The model under review builds one solid part; all positions refer to its coordinate system, in mm. A direction names the side the tool comes from. Give positions to 0.01 mm unless a question says otherwise; leave off trailing zeros. Write each loop counter-clockwise with the first axis right and the second up, starting at its lowest first coordinate (ties: lowest second). Pieces come first, ordered by that corner, then holes. Notation, with made-up numbers: M -37.75,-9 L -14.75,-9 A21 cw -14.75,30 Z; hole C -28,22.5 d1. An arc over 180 degrees is marked long. Write each question's results on one line, items separated by ' | '. Start each with the question number.
from build123d import *

# Parameters (mm, degrees)
SKETCH2_W           = 118
SKETCH2_H           = 80
BOSS_EXTRUDE1_DEPTH = 40
SKETCH3_R           = 12.5
BOSS_EXTRUDE2_DEPTH = 15


with BuildPart() as part:
    # Sketch2 → Boss-Extrude1 (new body)
    with BuildSketch(Plane(origin=(0, 0, 0), x_dir=(1, 0, 0), z_dir=(0, 1, 0))):
        with Locations((59, -40)):
            Rectangle(SKETCH2_W, SKETCH2_H)
    extrude(amount=BOSS_EXTRUDE1_DEPTH)

    # Sketch3 → Boss-Extrude2 (add)
    with BuildSketch(Plane(origin=(118, 0, 0), x_dir=(0, 0, -1), z_dir=(1, 0, 0))):
        with Locations((-55, 20)):
            Circle(SKETCH3_R)
        with Locations(Location((-25, 20, 0), (0, 0, 180))):
            Circle(SKETCH3_R)
    extrude(amount=BOSS_EXTRUDE2_DEPTH)


solid = part.part
(1) Draft analysis for pull direction Z (two halves, no side actions). For faces 1 (the flat face through (133, 20, 25)), 2 (the flat face through (58, 20, 0)), 3 (the cylindrical face through (125.395, 20.55, 67.488)), state which applies: pulls with the +Z half, pulls with the -Z half, needs draft (parallel to the pull), parting line crosses it, or undercut.
(2) Add section A-A (z = 55). State the section outline as (x, y) points.
(3) Machinability: for faces 4 (the cylindrical face through (125.395, 27.606, 15.08)), 5 (the flat face through (133, 20, 55)), which of the approach directions +Z, -Z, +X, -X, +Y, -Y give a long, thin tool a straight path to every point of the face, cutting with its end or side? Answer none if there is none.
(4) Wall thickness on L1, parallel to X at y = 7.5, z = 13; L2, parallel to Z at x = 127, y = 29.5; L3, parallel to Y at x = 120, z = 47: over which ranges is each line inside the solid? List them lowest first.
(5) Add section C-C (x = 123.5). State the section outline as (y, z) points, then the cut area to 3 significant figures.
(6) Add section D-D (y = 13.5). State the section outline as (x, z) points.
(7) Add section B-B (y = 20). State the section outline as (x, z) points, then the cut area to 3 significant figures.
Calculated:
1) face 1: needs draft | face 2: pulls with the -Z half | face 3: undercut
2) outline: M 0,0 L 118,0 L 118,7.5 L 133,7.5 L 133,32.5 L 118,32.5 L 118,40 L 0,40 Z
3) face 4: +X | face 5: +Z, -Z, +X, +Y, -Y
4) L1: x = 0 to 118 | L2: z = 16.88 to 33.12, 46.88 to 63.12 | L3: y = 10.4 to 29.6
5) outline: C 20,25 d25; C 20,55 d25 | area: 982 mm²
6) outline: M 0,0 L 118,0 L 118,14.32 L 133,14.32 L 133,35.68 L 118,35.68 L 118,44.32 L 133,44.32 L 133,65.68 L 118,65.68 L 118,80 L 0,80 Z
7) outline: M 0,0 L 118,0 L 118,12.5 L 133,12.5 L 133,37.5 L 118,37.5 L 118,42.5 L 133,42.5 L 133,67.5 L 118,67.5 L 118,80 L 0,80 Z | area: 10,200 mm²
